Part model, mm, in its own coordinate system. A direction names the side the tool comes from. Give positions to 0.01 mm unless a question says otherwise; leave off trailing zeros. Order: outer loops, then holes, each group sorted by start corner. A loop starts at its lowest first (then second) coordinate and runs counter-clockwise, first axis right, second up. Notation, with made-up numbers: M 34,-15.5 L 78,-15.5 A22 ccw 78,-2.5 Z; hole C -13,38 d7. An arc over 180 degrees is marked long. One line per question, with ' | ' between items.
```python
from build123d import *

# Parameters (mm, degrees)
CROQUIS1_R              = 5
CROQUIS1_R_2            = 7.55
SALIENTE_EXTRUIR1_DEPTH = 7
CROQUIS4_R              = 7.55
SALIENTE_EXTRUIR4_DEPTH = 52
CROQUIS5_R              = 4.1
CORTAR_EXTRUIR1_DEPTH   = 35
CROQUIS6_W              = 9.8
CROQUIS6_H              = 23
CORTAR_EXTRUIR2_DEPTH   = 41.5
CROQUIS7_R              = 1.4
CORTAR_EXTRUIR3_DEPTH   = 41.5
CROQUIS8_R              = 2.9
CROQUIS8_R_2            = 1.4
CORTAR_EXTRUIR4_DEPTH   = 3
CROQUIS10_R             = 1.5
CORTAR_EXTRUIR5_DEPTH   = 15
CROQUIS11_R             = 1.55
CORTAR_EXTRUIR6_DEPTH   = 60


with BuildPart() as part:
    # Croquis1 → Saliente-Extruir1 (new body)
    with BuildSketch(Plane(origin=(0, 0, 0), x_dir=(1, 0, 0), z_dir=(0, 1, 0))):
        with BuildLine():
            Line((28, 0), (28, 26))
            Line((28, 26), (-12.5, 26))
            Line((-12.5, 26), (-12.5, 0))
            ThreePointArc((-12.5, 0), (-4.303512587, -11.735833137), (9.536764706, -8.0808489))
            ThreePointArc((9.536764706, -8.0808489), (21.410465495, -10.077092543), (28, 0))
        make_face()
        Circle(CROQUIS1_R, mode=Mode.SUBTRACT)
        with Locations((17, 0)):
            Circle(CROQUIS1_R_2, mode=Mode.SUBTRACT)
    extrude(amount=SALIENTE_EXTRUIR1_DEPTH)

    # Croquis4 → Saliente-Extruir4 (add)
    with BuildSketch(Plane.XZ):
        with BuildLine():
            Line((-12.5, -12), (-12.5, -26))
            Line((-12.5, -26), (28, -26))
            Line((28, -26), (28, 0))
            ThreePointArc((28, 0), (21.410465495, 10.077092543), (9.536764706, 8.0808489))
            ThreePointArc((9.536764706, 8.0808489), (6.922907457, 4.410465495), (6, 0))
            Line((6, 0), (6, -12))
            Line((6, -12), (-12.5, -12))
        make_face()
        with Locations((17, 0)):
            Circle(CROQUIS4_R, mode=Mode.SUBTRACT)
    extrude(amount=SALIENTE_EXTRUIR4_DEPTH)

    # Croquis5 → Cortar-Extruir1 (cut)
    with BuildSketch(Plane.ZY.offset(12.5)):
        with Locations((-19.25, -1)):
            Circle(CROQUIS5_R)
        with Locations((-19.25, -46)):
            Circle(CROQUIS5_R)
    extrude(amount=-CORTAR_EXTRUIR1_DEPTH, mode=Mode.SUBTRACT)

    # Croquis6 → Cortar-Extruir2 (cut, through all)
    with BuildSketch(Plane.ZY.offset(12.5)):
        with Locations((-19.25, -23.5)):
            Rectangle(CROQUIS6_W, CROQUIS6_H)
    extrude(amount=-CORTAR_EXTRUIR2_DEPTH, mode=Mode.SUBTRACT)

    # Croquis7 → Cortar-Extruir3 (cut, through all)
    with BuildSketch(Plane(origin=(28, 0, 0), x_dir=(0, 0, -1), z_dir=(1, 0, 0))):
        with Locations((19.25, -1)):
            Circle(CROQUIS7_R)
        with Locations((19.25, -46)):
            Circle(CROQUIS7_R)
    extrude(amount=-CORTAR_EXTRUIR3_DEPTH, mode=Mode.SUBTRACT)

    # Croquis8 → Cortar-Extruir4 (cut)
    with BuildSketch(Plane(origin=(28, 0, 0), x_dir=(0, 0, -1), z_dir=(1, 0, 0))):
        with Locations((19.25, -1)):
            Circle(CROQUIS8_R)
        with Locations((19.25, -1)):
            Circle(CROQUIS8_R_2, mode=Mode.SUBTRACT)
        with Locations((19.25, -46)):
            Circle(CROQUIS8_R)
        with Locations((19.25, -46)):
            Circle(CROQUIS8_R_2, mode=Mode.SUBTRACT)
    extrude(amount=-CORTAR_EXTRUIR4_DEPTH, mode=Mode.SUBTRACT)

    # Croquis10 → Cortar-Extruir5 (cut, through all)
    with BuildSketch(Plane.XY.offset(-12)):
        with Locations((-5.5, -23.5)):
            Circle(CROQUIS10_R)
    extrude(amount=-CORTAR_EXTRUIR5_DEPTH, mode=Mode.SUBTRACT)

    # Croquis11 → Cortar-Extruir6 (cut, through all)
    with BuildSketch(Plane(origin=(0, 7, 0), x_dir=(1, 0, 0), z_dir=(0, 1, 0))):
        with Locations((0, 8)):
            Circle(CROQUIS11_R)
        with Locations((0, -8)):
            Circle(CROQUIS11_R)
    extrude(amount=-CORTAR_EXTRUIR6_DEPTH, mode=Mode.SUBTRACT)


solid = part.part
```
1. Drop flat-ended pins along their axis: pin 1 (6 mm diameter, centred on y = -13, z = 2.5, fed in from -X); pin 2 (2 mm diameter, centred on y = 0.5, z = -20, fed in from +X); pin 3 (11 mm diameter, centred on x = -0.5, z = -5, fed in from -Y). Give the stop position or say it passes through.
Worked out:
pin 1: stops at x = 6 | pin 2: stops at x = 25 | pin 3: stops at y = 0
2. Mould opens along X. For faces 6 (the flat face through (7, -24, -24.15)), 7 (the cylindrical face through (9.457, -22.087, 0.332)), 8 (the flat face through (22.5, -3, -19)) say: released by +X, released by -X, zero draft, split by the parting line, or undercut.
Worked out:
face 6: zero draft | face 7: undercut | face 8: released by -X
3. Slice it at C-C on y = -23.5. Give the cut face in (x, z), then the cut area to 3 significant figures.
Worked out:
outline: M -12.5,-26 L -7,-26 L -7,-24.15 L -12.5,-24.15 Z; M -12.5,-14.35 L -7,-14.35 L -7,-12 L -12.5,-12 Z; M -4,-26 L 28,-26 L 28,-24.15 L -4,-24.15 Z; M -4,-14.35 L 28,-14.35 L 28,0 A11 ccw 6,0 L 6,-12 L -4,-12 Z; hole C 17,0 d15.1 | area: 432 mm2
4. Tool access for faces 1 (the cylindrical face through (4.755, -45.82, -23.346)), 2 (the flat face through (-7, 0, 0)), 3 (the cylindrical face through (-6.61, -22.49, -13.16)), 4 (the flat face through (25, -2, -18)), 5 (the flat face through (7, -12, -19)): list every direction of +Z, -Z, +X, -X, +Y, -Y with a clear straight run to the whole face (end or side of a thin tool).
Worked out:
face 1: -X | face 2: +Z, -X, -Y | face 3: +Z, -Z | face 4: +X | face 5: +X, -X
5. Slice it at A-A on y = -1. Give the cut face in (x, z), then the cut area to 3 significant figures.
Worked out:
outline: M -12.5,-26 L 28,-26 L 28,-22.15 L 25,-22.15 L 25,-20.65 L 22.5,-20.65 L 22.5,-23.35 L -12.5,-23.35 Z; M -12.5,-15.15 L 22.5,-15.15 L 22.5,-17.85 L 25,-17.85 L 25,-16.35 L 28,-16.35 L 28,0 A11 ccw 6,0 L 6,-12 L -12.5,-12 Z; hole C 17,0 d15.1 | area: 531 mm2
6. Slice it at D-D on x = 16. Give the cut face in (y, z), then the cut area to 3 significant figures.
Worked out:
outline: M -52,-26 L 7,-26 L 7,-7.48 L -52,-7.48 Z; M -52,7.48 L 7,7.48 L 7,10.95 L -52,10.95 Z; hole C -46,-19.25 d8.2; hole M -35,-24.15 L -12,-24.15 L -12,-14.35 L -35,-14.35 Z; hole C -1,-19.25 d8.2 | area: 966 mm2
7. Slice it at B-B on x = 0. Give the cut face in (y, z).
Worked out:
outline: M -52,-26 L 7,-26 L 7,-9.55 L 0,-9.55 L 0,-12 L -52,-12 Z; M 0,-6.45 L 7,-6.45 L 7,-5 L 0,-5 Z; M 0,5 L 7,5 L 7,6.45 L 0,6.45 Z; M 0,9.55 L 7,9.55 L 7,12.5 L 0,12.5 Z; hole C -46,-19.25 d8.2; hole M -35,-24.15 L -12,-24.15 L -12,-14.35 L -35,-14.35 Z; hole C -1,-19.25 d8.2
8. Probe L1, parallel to X at y = -13.5, z = 0; L2, parallel to Y at x = 23, z = -19; L3, parallel to Y at x = 2.5, z = -24. List the from-to ranges inside material, lowest first. Write a range as from..to.
Worked out:
L1: x = 6..9.45, 24.55..28 | L2: y = -52..-47.38, -44.62..-35, -12..-2.38, 0.38..7 | L3: y = -52..-35, -12..7
